Could you check a few things on this drawing? It's one solid part, dimensions in mm from its lowest x, y, z. A direction names the side the tool comes from. Round coordinates to 2 decimals unless told otherwise and drop trailing zeros. Loops run counter-clockwise (first coordinate to the right, second up) from the corner with the lowest first, then second, coordinate; pieces in that order, holes last. Notation, with made-up numbers: M -27.75,-22.5 L 25.25,-22.5 A24 cw 25.25,1.5 Z; hole C -32,43 d9. An arc over 180 degrees is marked long. Answer as a JSON object with one key per item and string values.
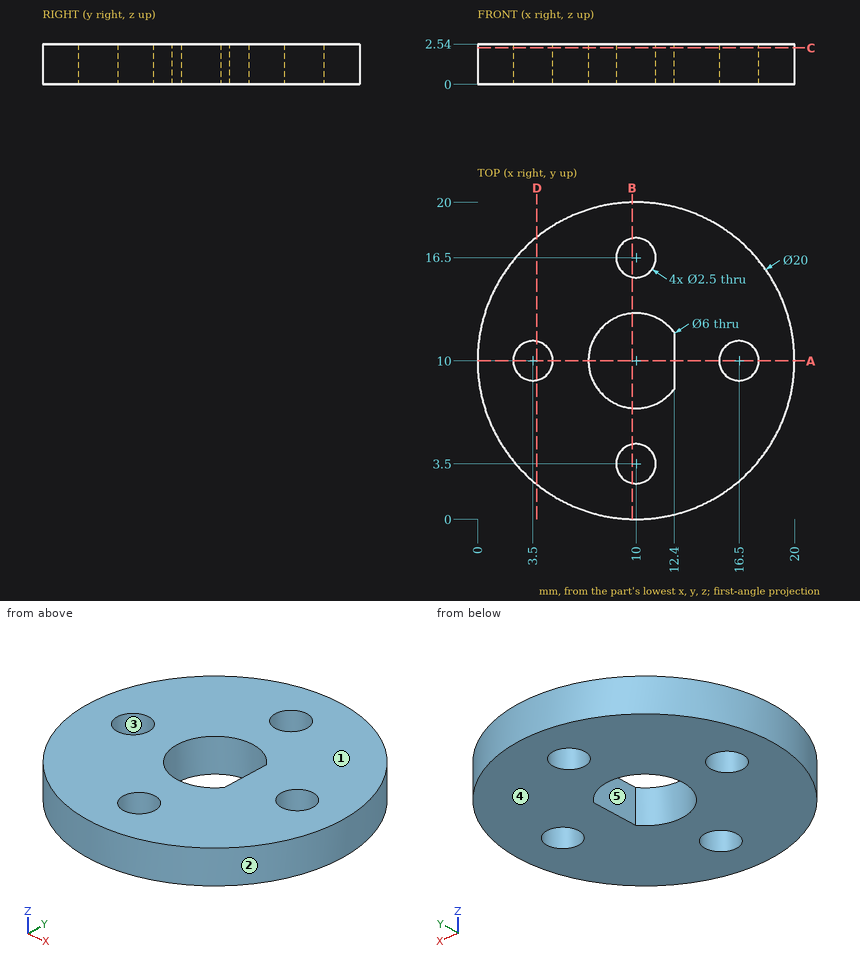
Item 1: If we mould it in two halves opening along Y, with no side actions, what happens to the marked faces 1, 2 and 3? For each: pulls with the +Y half, pulls with the -Y half, needs draft (parallel to the pull), parting line crosses it, or undercut.
Resolved:
{"face 1": "needs draft", "face 2": "parting line crosses it", "face 3": "undercut"}
Item 2: I'm going to push flat-ended pins straight in: pin 1 Ø1.5 at (y, z) = (17, 1) entering from -X; pin 2 Ø1.5 at (x, y) = (10, 3.5) entering from -Z; pin 3 Ø1.5 at (y, z) = (16, 2) entering from -X. Where does each tip first touch, or does it pass through?
Resolved:
{"pin 1": "x = 2.19", "pin 2": "through", "pin 3": "x = 1.49"}
Item 3: I want a section at A-A, the plane y = 10. Please give me the cut outline in (x, z), then the cut area to 3 significant figures.
Resolved:
{"outline": "M 0,0 L 2.25,0 L 2.25,2.54 L 0,2.54 Z; M 4.75,0 L 7,0 L 7,2.54 L 4.75,2.54 Z; M 12.4,0 L 15.25,0 L 15.25,2.54 L 12.4,2.54 Z; M 17.75,0 L 20,0 L 20,2.54 L 17.75,2.54 Z", "area": "24.4 mm²"}
Item 4: On a 3-axis mill with a long thin cutter (end or side, diameter ignored), from which of +Z, -Z, +X, -X, +Y, -Y can I reach the whole of each face in a straight line? I mean the marked faces 4 and 5. Say none if no direction works.
Resolved:
{"face 4": "-Z, +X, -X, +Y, -Y", "face 5": "+Z, -Z"}
Item 5: I want a section at C-C, the plane z = 2.3. Please give me the cut outline in (x, y), then the cut area to 3 significant figures.
Resolved:
{"outline": "C 10,10 d20; hole C 3.5,10 d2.5; hole C 10,3.5 d2.5; hole C 10,16.5 d2.5; hole M 12.4,8.2 L 12.4,11.8 A3 ccw long Z; hole C 16.5,10 d2.5", "area": "268 mm²"}
Item 6: Please list where these lines run through material, in increasing order: probe 1 along Y at (x, z) = (10, 1.45); probe 2 along Y at (x, z) = (10.5, 2.15); probe 3 along X at (y, z) = (17, 2.15). Write a range as from..to.
Resolved:
{"probe 1": "0..2.25, 4.75..7, 13..15.25, 17.75..20", "probe 2": "0.01..2.35, 4.65..7.04, 12.96..15.35, 17.65..19.99", "probe 3": "2.86..8.85, 11.15..17.14"}
Item 7: I want a section at D-D, the plane x = 3.75. Please give me the cut outline in (y, z), then the cut area to 3 significant figures.
Resolved:
{"outline": "M 2.19,0 L 8.78,0 L 8.78,2.54 L 2.19,2.54 Z; M 11.22,0 L 17.81,0 L 17.81,2.54 L 11.22,2.54 Z", "area": "33.4 mm²"}
Item 8: I want a section at B-B, the plane x = 9.75. Please give me the cut outline in (y, z).
Resolved:
{"outline": "M 0,0 L 2.28,0 L 2.28,2.54 L 0,2.54 Z; M 4.72,0 L 7.01,0 L 7.01,2.54 L 4.72,2.54 Z; M 12.99,0 L 15.28,0 L 15.28,2.54 L 12.99,2.54 Z; M 17.72,0 L 20,0 L 20,2.54 L 17.72,2.54 Z"}
